Design review of the part built by this model. Coordinates are the model's own, in mm. A direction names the side the tool comes from. Coordinates: 2 decimals unless noted, no trailing zeros. Loops run counter-clockwise (first coordinate to the right, second up) from the corner with the lowest first, then second, coordinate; pieces in that order, holes last.
Q1. Draft analysis for pull direction X (two halves, no side actions). For faces 5 (the face through (-2, -12, 6)), 6 (the face through (-1.1, -0.1, 3)), 7 (the face through (2, -13, 3)), state which applies: released by +X, released by -X, zero draft, split by the parting line, or undercut.
Q2. Wall thickness on probe 1 along Y at (x, z) = (0.25, 3.75); probe 2 along Y at (x, z) = (1.5, 2.75); probe 3 along X at (y, z) = (-3.5, 5.5): over which ranges is each line inside the solid? List them lowest first.
Q3. For P1, Ø4.5, axis at x = -0.5, y = -5, coming from the +Z side; P2, Ø2, axis at x = 2.5, z = 7.5, coming from the +Y side; P3, Ø1.5, axis at x = 0, y = -1.5, coming from the +Z side, all flat-tipped, find the tip position at first contact; note any pin that passes through.
Q4. Add section D-D on x = -3.5. Give the boundary of the cut face in (y, z).
Q5. Machinability: for faces 1 (the face through (-2, 13, 6)), 2 (the face through (-1.3, 0, 6)), 3 (the face through (-5, 0, 7)), 4 (the face through (1, 14.35, 3)), which of the approach directions +Z, -Z, +X, -X, +Y, -Y give a long, thin tool a straight path to every point of the face, cutting with its end or side? Answer none if there is none.
Q6. Add section A-A on y = -12.5. Give the boundary of the cut face in (x, z).
Q7. Add section C-C on z = 2. Give the boundary of the cut face in (x, y).
Q8. Add section B-B on x = 3. Give the boundary of the cut face in (y, z).
```python
from build123d import *

# Parameters (mm, degrees)
SKETCH_1_W          = 2
SKETCH_1_H          = 3
EXTRUDE_1_DEPTH     = 6
EXTRUDE_2_DEPTH     = 3
SKETCH_3_W          = 1
SKETCH_3_H          = 34.7
CUT_EXTRUDE_1_DEPTH = 9


with BuildPart() as part:
    # 草圖1 → 填料-伸長1 (new body)
    with BuildSketch(Plane.XY):
        with BuildLine():
            Line((5, 17.35), (-5, 17.35))
            Line((-5, 17.35), (-5, -17.35))
            Line((-5, -17.35), (5, -17.35))
            Line((5, -17.35), (5, -6.1))
            ThreePointArc((5, -6.1), (-1.1, 0), (5, 6.1))
            Line((5, 6.1), (5, 17.35))
        make_face()
        with Locations((1, -12.85)):
            Rectangle(SKETCH_1_W, SKETCH_1_H, mode=Mode.SUBTRACT)
        with Locations((1, 12.85)):
            Rectangle(SKETCH_1_W, SKETCH_1_H, mode=Mode.SUBTRACT)
    extrude(amount=EXTRUDE_1_DEPTH)

    # 草圖2 → 填料-伸長2 (add)
    with BuildSketch(Plane.XY.offset(6)):
        with BuildLine():
            Line((5, 10), (5, 8))
            ThreePointArc((5, 8), (-3, 0), (5, -8))
            Line((5, -8), (5, -10))
            ThreePointArc((5, -10), (-5, 0), (5, 10))
        make_face()
    extrude(amount=EXTRUDE_2_DEPTH)

    # 草圖3 → 除料-伸長1 (cut, symmetric)
    with BuildSketch(Plane.XY.offset(6)):
        with Locations((4.5, 0)):
            Rectangle(SKETCH_3_W, SKETCH_3_H)
    extrude(amount=CUT_EXTRUDE_1_DEPTH, both=True, mode=Mode.SUBTRACT)


solid = part.part
```
Entries:
1. face 5: zero draft
1. face 6: released by +X
1. face 7: undercut
2. probe 1: y = -17.35 to -14.35, -11.35 to -3.83, 3.83 to 11.35, 14.35 to 17.35
2. probe 2: y = -17.35 to -14.35, -11.35 to -5, 5 to 11.35, 14.35 to 17.35
2. probe 3: x = -5 to 0
3. P1: stops at z = 9
3. P2: stops at y = 9.89
3. P3: passes through
4. outline: (-17.35, 0) - (17.35, 0) - (17.35, 6) - (5.27, 6) - (5.27, 9) - (-5.27, 9) - (-5.27, 6) - (-17.35, 6) - close
5. face 1: +Z, -X, +Y
5. face 2: +Z, +X
5. face 3: +Z, -X
5. face 4: +Z, -Z
6. outline: (-5, 0) - (0, 0) - (0, 6) - (-5, 6) - close; (2, 0) - (4, 0) - (4, 6) - (2, 6) - close
7. outline: (-5, -17.35) - (4, -17.35) - (4, -6.02) arc R6.1 cw to (4, 6.02) - (4, 17.35) - (-5, 17.35) - close; hole (0, -14.35) - (2, -14.35) - (2, -11.35) - (0, -11.35) - close; hole (0, 11.35) - (2, 11.35) - (2, 14.35) - (0, 14.35) - close
8. outline: (-17.35, 0) - (-5.76, 0) - (-5.76, 6) - (-7.75, 6) - (-7.75, 9) - (-9.8, 9) - (-9.8, 6) - (-17.35, 6) - close; (5.76, 0) - (17.35, 0) - (17.35, 6) - (9.8, 6) - (9.8, 9) - (7.75, 9) - (7.75, 6) - (5.76, 6) - close
